```python
from build123d import *

# Parameters (mm, degrees)
SKETCH_1_W          = 50
SKETCH_1_H          = 100
EXTRUDE_1_DEPTH     = 10
EXTRUDE_START       = -36
EXTRUDE_2_DEPTH     = 36
SKETCH_2_W          = 50
SKETCH_2_H          = 10
EXTRUDE_3_DEPTH     = 51
SKETCH_3_R          = 7.5
CUT_EXTRUDE_1_DEPTH = 116.004347744
EXTRUDE_4_DEPTH     = 6


with BuildPart() as part:
    # Sketch 1 → Extrude 1 (new body)
    # profile 1 of 2: a face of its own
    with BuildSketch(Plane.XY):
        Rectangle(SKETCH_1_W, SKETCH_1_H)
        with BuildLine():
            ThreePointArc((-16, -20), (0, -36), (16, -20))
            Line((16, -20), (16, 20))
            ThreePointArc((16, 20), (0, 36), (-16, 20))
            Line((-16, 20), (-16, -20))
        make_face(mode=Mode.SUBTRACT)
    # profile 2 of 2: a face of its own
    with BuildSketch(Plane.XY):
        with BuildLine():
            Line((-16, -20), (-16, 20))
            ThreePointArc((-16, 20), (0, 36), (16, 20))
            Line((16, 20), (16, -20))
            ThreePointArc((16, -20), (0, -36), (-16, -20))
        make_face()
        with BuildLine():
            ThreePointArc((6, 20), (0, 26), (-6, 20))
            Line((-6, 20), (-6, -20))
            ThreePointArc((-6, -20), (0, -26), (6, -20))
            Line((6, -20), (6, 20))
        make_face(mode=Mode.SUBTRACT)
    extrude(amount=EXTRUDE_1_DEPTH)

    # Sketch 1_3 → Extrude 2 (add)
    with BuildSketch(Plane.XY.offset(EXTRUDE_START)):
        with BuildLine():
            Line((-16, -20), (-16, 20))
            ThreePointArc((-16, 20), (0, 36), (16, 20))
            Line((16, 20), (16, -20))
            ThreePointArc((16, -20), (0, -36), (-16, -20))
        make_face()
        with BuildLine():
            ThreePointArc((6, 20), (0, 26), (-6, 20))
            Line((-6, 20), (-6, -20))
            ThreePointArc((-6, -20), (0, -26), (6, -20))
            Line((6, -20), (6, 20))
        make_face(mode=Mode.SUBTRACT)
    extrude(amount=EXTRUDE_2_DEPTH)

    # Sketch 2 → Extrude 3 (add)
    with BuildSketch(Plane(origin=(0, 0, 0), x_dir=(-1, 0, 0), z_dir=(0, 0, -1))):
        with Locations((0, 55)):
            Rectangle(SKETCH_2_W, SKETCH_2_H)
    extrude(amount=-EXTRUDE_3_DEPTH)

    # Sketch 3 → Cut-Extrude 1 (cut, through all)
    with BuildSketch(Plane.XZ.offset(-50)):
        with Locations(Location((0, 30.5, 0), (0, 0, 270))):
            Circle(SKETCH_3_R)
    extrude(amount=-CUT_EXTRUDE_1_DEPTH, mode=Mode.SUBTRACT)

    # Sketch 4 → Extrude 4 (add)
    with BuildSketch(Plane.ZY.offset(25)):
        Polygon((51, 50), (10, -50), (10, 50), align=None)
    extrude(amount=-EXTRUDE_4_DEPTH)


solid = part.part
```
Verification items for the finished model (mm, model axes). A direction names the side the tool comes from. Coordinates: 2 decimals unless noted, no trailing zeros. Loops run counter-clockwise (first coordinate to the right, second up) from the corner with the lowest first, then second, coordinate; pieces in that order, holes last. Notation, with made-up numbers: (36.5, 13.25) - (68.5, 13.25) arc R21 ccw to (68.5, 45.25) - close; hole circle Ø1 at (40.5, 47). An arc over 180 degrees is marked (long way). Return JSON: item names as keys, results as strings.
1. Mould release check, pull along Y, two halves, no side actions. Record for faces 1 (the flat face through (17, 6, 0)), 2 (the flat face through (0, -50, 5)), 3 (the flat face through (-6, 0, -13)), 4 (the cylindrical face through (0, 26, -13)): +Y half, -Y half, draft (parallel to the pull), parting line (faces both ways), or undercut.
Established:
{"face 1": "draft", "face 2": "-Y half", "face 3": "undercut", "face 4": "undercut"}
2. Thickness scan on L1, parallel to X at y = 55, z = 30; L2, parallel to Y at x = -15.5, z = 27; L3, parallel to Z at x = 9, y = -14. Record the ranges inside material, lowest first.
Established:
{"L1": "x = -25 to -7.48, 7.48 to 25", "L2": "y = 50 to 60", "L3": "z = -36 to 10"}
3. Section check C-C, the plane z = 30.5. Record the boundary of the cut face in (x, y).
Established:
{"outline": "(-25, 0) - (-19, 0) - (-19, 50) - (-7.5, 50) - (-7.5, 60) - (-25, 60) - close; (7.5, 50) - (25, 50) - (25, 60) - (7.5, 60) - close"}
4. Section check D-D, the plane z = -8. Record the boundary of the cut face in (x, y).
Established:
{"outline": "(-16, -20) arc R16 ccw to (16, -20) - (16, 20) arc R16 ccw to (-16, 20) - close; hole (-6, -20) arc R6 ccw to (6, -20) - (6, 20) arc R6 ccw to (-6, 20) - close"}
5. Go/stop test with flat-tipped pins: pin 1 (20 mm diameter, centred on y = -1, z = -21, fed in from -X); pin 2 (12.5 mm diameter, centred on x = 0, z = 37.5, fed in from -Y); pin 3 (2 mm diameter, centred on x = 15.5, y = 28, fed in from -Z); pin 4 (8 mm diameter, centred on x = 12.5, z = 11.5, fed in from -Y). Record where each tip stops, or that it passes through.
Established:
{"pin 1": "stops at x = -16", "pin 2": "stops at y = 50", "pin 3": "stops at z = 0", "pin 4": "stops at y = -50"}
6. Section check A-A, the plane y = -16. Record the boundary of the cut face in (x, z), then the cut area to 3 significant figures.
Established:
{"outline": "(-25, 0) - (-16, 0) - (-16, -36) - (-6, -36) - (-6, 10) - (-19, 10) - (-19, 23.94) - (-25, 23.94) - close; (6, -36) - (16, -36) - (16, 0) - (25, 0) - (25, 10) - (6, 10) - close", "area": "1,180 mm2"}
7. Tool access check on faces 5 (the flat face through (16, 0, -18)), 6 (the cylindrical face through (0, 36, -18)), 7 (the flat face through (6, 0, -13)). Record the directions out of +Z, -Z, +X, -X, +Y, -Y that give a thin tool (end or side, any length) a straight path to the whole face; none if there is none.
Established:
{"face 5": "-Z, +X, +Y, -Y", "face 6": "-Z, +Y", "face 7": "+Z, -Z"}
8. Section check B-B, the plane x = 0. Record the boundary of the cut face in (y, z).
Established:
{"outline": "(-50, 0) - (-36, 0) - (-36, -36) - (-26, -36) - (-26, 10) - (-50, 10) - close; (26, -36) - (36, -36) - (36, 0) - (60, 0) - (60, 23) - (50, 23) - (50, 10) - (26, 10) - close; (50, 38) - (60, 38) - (60, 51) - (50, 51) - close"}
